Study the drawing (mm; zero at the part's minimum x, y, z) and answer. A direction names the side the tool comes from. Round coordinates to 2 decimals unless told otherwise and drop trailing zeros. Loops run counter-clockwise (first coordinate to the right, second up) from the corner with the lowest first, then second, coordinate; pieces in that order, holes last. Notation, with made-up numbers: (76.25, 22) - (116.25, 22) arc R8 ccw to (116.25, 37) - close; hole circle Ø8 at (28.25, 25). An arc over 180 degrees is marked (long way). One line per item, written item: value.
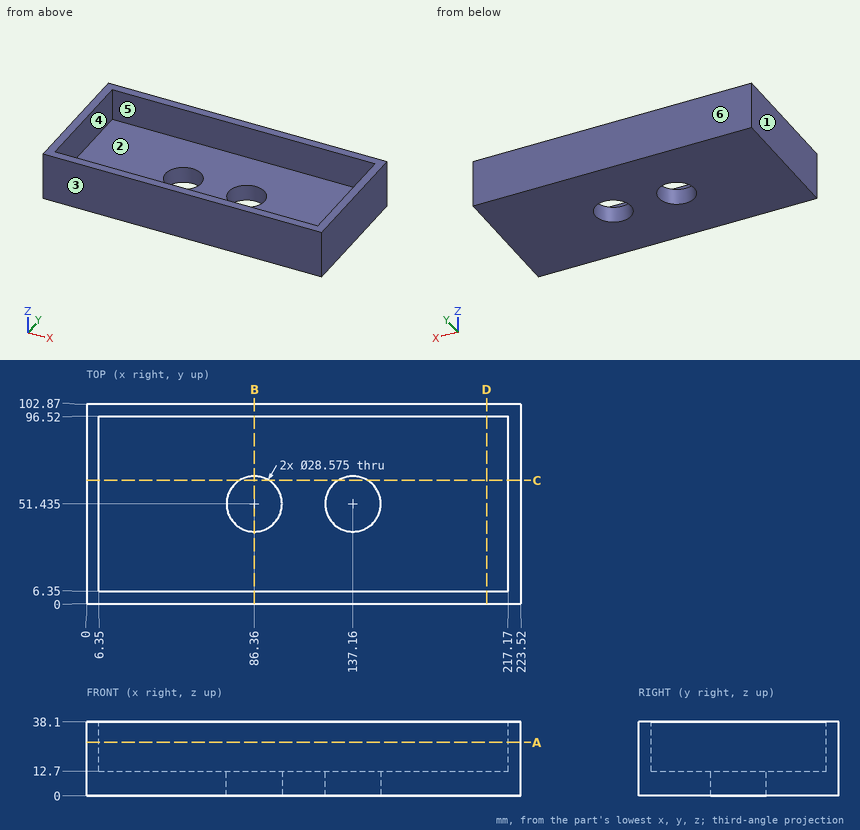
1) This flat-tipped pin is pushed along its axis until it touches: pin 1 Ø6 at (y, z) = (10.5, 28.5) entering from -X. Where does it stop, or does it pass through?
Final values:
pin 1: x = 0
2) For the marked faces 1 and 2, determine the directions among +Z, -Z, +X, -X, +Y, -Y from which every point of the face is accessible in a straight line to the end or side of a thin tool.
Final values:
face 1: +Z, -Z, -X, +Y, -Y
face 2: +Z
3) Consider L1, parallel to Y at x = 137.16, z = 6.75; L2, parallel to X at y = 33.5, z = 18.5; L3, parallel to Y at x = 132, z = 14. Determine where each line is inside the solid, lowest interval first.
Final values:
L1: 0 to 37.15, 65.72 to 102.87
L2: 0 to 6.35, 217.17 to 223.52
L3: 0 to 6.35, 96.52 to 102.87
4) A cutting plane is placed at D-D on x = 206. Give the vertices of the cut face in (y, z).
Final values:
outline: (0, 0) - (102.87, 0) - (102.87, 38.1) - (96.52, 38.1) - (96.52, 12.7) - (6.35, 12.7) - (6.35, 38.1) - (0, 38.1) - close
5) For a pull along Y with two mould halves and no side action, classify the marked faces 3, 4, 5 and 6 as released by +Y, released by -Y, zero draft, split by the parting line, or undercut.
Final values:
face 3: released by -Y
face 4: undercut
face 5: undercut
face 6: released by +Y
6) A cutting plane is placed at A-A on z = 27.5. Give the vertices of the cut face in (x, y).
Final values:
outline: (0, 0) - (223.52, 0) - (223.52, 102.87) - (0, 102.87) - close; hole (6.35, 6.35) - (217.17, 6.35) - (217.17, 96.52) - (6.35, 96.52) - close
7) A cutting plane is placed at C-C on y = 63.5. Give the vertices of the cut face in (x, z).
Final values:
outline: (0, 0) - (78.71, 0) - (78.71, 12.7) - (6.35, 12.7) - (6.35, 38.1) - (0, 38.1) - close; (94.01, 0) - (129.51, 0) - (129.51, 12.7) - (94.01, 12.7) - close; (144.81, 0) - (223.52, 0) - (223.52, 38.1) - (217.17, 38.1) - (217.17, 12.7) - (144.81, 12.7) - close
8) A cutting plane is placed at B-B on x = 86.36. Give the vertices of the cut face in (y, z), and give its area (3 significant figures).
Final values:
outline: (0, 0) - (37.15, 0) - (37.15, 12.7) - (6.35, 12.7) - (6.35, 38.1) - (0, 38.1) - close; (65.72, 0) - (102.87, 0) - (102.87, 38.1) - (96.52, 38.1) - (96.52, 12.7) - (65.72, 12.7) - close
area: 1,270 mm2
